Verification items for the finished model (mm, model axes). A direction names the side the tool comes from. Round coordinates to 2 decimals unless told otherwise and drop trailing zeros. Put each result on its own line as item: value.
```python
from build123d import *

# Parameters (mm, degrees)
ESQUISSE1_RX            = 12.5
ESQUISSE1_RY            = 12.5
BOSS_EXTRU_1_DEPTH      = 6
ESQUISSE2_R             = 5
ENL_V_MAT_EXTRU_1_DEPTH = 4
ENL_V_MAT_EXTRU_2_REACH = 20.125
ESQUISSE3_R             = 3.75
CHANFREIN1_SIZE         = 0.5
ENL_V_MAT_EXTRU_3_DEPTH = 4
ENL_V_MAT_EXTRU_4_REACH = 20.125
ESQUISSE6_R             = 1.7


with BuildPart() as part:
    # Esquisse1 → Boss.-Extru.1 (new body)
    with BuildSketch(Plane.XY):
        with Locations((0, 0)):
            Ellipse(ESQUISSE1_RX, ESQUISSE1_RY)
    extrude(amount=BOSS_EXTRU_1_DEPTH)

    # Esquisse2 → Enlèv. mat.-Extru.1 (cut)
    with BuildSketch(Plane(origin=(0, 0, 0), x_dir=(-1, 0, 0), z_dir=(0, 0, -1))):
        Circle(ESQUISSE2_R)
    extrude(amount=-ENL_V_MAT_EXTRU_1_DEPTH, mode=Mode.SUBTRACT)

    # Esquisse3 → Enlèv. mat.-Extru.2 (cut, up to next)
    with BuildSketch(Plane(origin=(0, 0, 4), x_dir=(-1, 0, 0), z_dir=(0, 0, -1)), mode=Mode.PRIVATE) as enl_v_mat_extru_2_sk1:
        Circle(ESQUISSE3_R)
    enl_v_mat_extru_2_tool1 = extrude(enl_v_mat_extru_2_sk1.sketch, amount=-ENL_V_MAT_EXTRU_2_REACH, mode=Mode.PRIVATE) & part.part
    add(enl_v_mat_extru_2_tool1.solids().sort_by_distance((0, 0, 4))[0], mode=Mode.SUBTRACT)

    # Chanfrein1
    chanfrein1_edges = [part.edges().sort_by_distance(p)[0] for p in [
        (3.75, 0, 4),
    ]]
    chamfer(chanfrein1_edges, length=CHANFREIN1_SIZE)

    # Esquisse5 → Enlèv. mat.-Extru.3 (cut)
    with BuildSketch(Plane(origin=(0, 0, 0), x_dir=(-1, 0, 0), z_dir=(0, 0, -1))):
        Polygon((-3.117691454, -8.75), (-1.558845727, -11.45), (1.558845727, -11.45), (3.117691454, -8.75), (1.558845727, -6.05), (-1.558845727, -6.05), align=None)
        Polygon((3.117691454, 8.75), (1.558845727, 11.45), (-1.558845727, 11.45), (-3.117691454, 8.75), (-1.558845727, 6.05), (1.558845727, 6.05), align=None)
    extrude(amount=-ENL_V_MAT_EXTRU_3_DEPTH, mode=Mode.SUBTRACT)

    # Esquisse6 → Enlèv. mat.-Extru.4 (cut, up to next)
    with BuildSketch(Plane(origin=(0, 0, 4), x_dir=(-1, 0, 0), z_dir=(0, 0, -1)), mode=Mode.PRIVATE) as enl_v_mat_extru_4_sk1:
        with Locations((0, 8.75)):
            Circle(ESQUISSE6_R)
    enl_v_mat_extru_4_tool1 = extrude(enl_v_mat_extru_4_sk1.sketch, amount=-ENL_V_MAT_EXTRU_4_REACH, mode=Mode.PRIVATE) & part.part
    # Esquisse6 → Enlèv. mat.-Extru.4 (cut, up to next)
    with BuildSketch(Plane(origin=(0, 0, 4), x_dir=(-1, 0, 0), z_dir=(0, 0, -1)), mode=Mode.PRIVATE) as enl_v_mat_extru_4_sk2:
        with Locations((0, -8.75)):
            Circle(ESQUISSE6_R)
    enl_v_mat_extru_4_tool2 = extrude(enl_v_mat_extru_4_sk2.sketch, amount=-ENL_V_MAT_EXTRU_4_REACH, mode=Mode.PRIVATE) & part.part
    add(enl_v_mat_extru_4_tool1.solids().sort_by_distance((0, 8.75, 4))[0], mode=Mode.SUBTRACT)
    add(enl_v_mat_extru_4_tool2.solids().sort_by_distance((0, -8.75, 4))[0], mode=Mode.SUBTRACT)


solid = part.part
```
Item 1: Depth check by flat-ended pin: pin 1 Ø1.5 at (y, z) = (1, 3.5) entering from +X; pin 2 Ø2.5 at (x, y) = (1, 9.5) entering from -Z; pin 3 Ø1.5 at (x, z) = (10, 2.5) entering from +Y. Enter the tip coordinate at first touch or a pass-through.
Geometry check:
pin 1: x = 12.5
pin 2: z = 4
pin 3: y = 8.41
Item 2: Release check for a two-part mould opening along Y. For faces 1 (the face through (3, 3, 6)), 2 (the face through (0, -6.05, 2)) record: pulls with the +Y half, pulls with the -Y half, needs draft (parallel to the pull), parting line crosses it, or undercut.
Geometry check:
face 1: needs draft
face 2: undercut
Item 3: Sectioned sample at A-A, the plane x = 0. Give the number of separate pieces and of enclosed holes in the cut face, then the cut area to 4 significant figures.
Geometry check:
separate pieces: 4
enclosed holes: 0
area: 37.95 mm2
Item 4: Material ranges on line 1 along Y through (x, z) = (0, 5.05); line 2 along Y through (x, z) = (0, 2.05); line 3 along Z through (x, y) = (1.5, -11.25), recorded low to high.
Geometry check:
line 1: -12.5 to -10.45, -7.05 to -3.75, 3.75 to 7.05, 10.45 to 12.5
line 2: -12.5 to -11.45, -6.05 to -5, 5 to 6.05, 11.45 to 12.5
line 3: 4 to 6
Item 5: Tool access check on faces 3 (the face through (0.37, -10.41, 4.99)), 4 (the face through (-2.35, -7.42, 1.97)). Record the directions out of +Z, -Z, +X, -X, +Y, -Y that give a thin tool (end or side, any length) a straight path to the whole face; none if there is none.
Geometry check:
face 3: +Z, -Z
face 4: -Z
